from build123d import *

# Parameters (mm, degrees)
F0_W     = 1.6
F0_H     = 10
F1_DEPTH = 8
F2_R     = 2
F3_SIZE  = 3


with BuildPart() as f1:
    # F0 (on Top) → F1 (new body)
    with BuildSketch(Plane.XY):
        Polygon((9.2, 5.6), (9.2, 3.6), (11.2, 5.6), align=None)
        Polygon((7.6, 0), (9.2, 0), (9.2, 3.6), (9.2, 5.6), (9.2, 17.6), (7.6, 17.6), align=None)
        with BuildLine():
            Line((1.6, 0), (0, 0))
            ThreePointArc((0, 0), (4.6, -4.6), (9.2, 0))
            Line((9.2, 0), (7.6, 0))
            ThreePointArc((7.6, 0), (4.6, -3), (1.6, 0))
        make_face()
        with Locations((0.8, 5)):
            Rectangle(F0_W, F0_H)
        Polygon((-8.4, 10), (0, 10), (1.6, 10), (1.6, 11.6), (-8.4, 11.6), align=None)
    extrude(amount=F1_DEPTH)

    # F2
    f2_edges = [f1.edges().sort_by_distance(p)[0] for p in [
        (9.2, 3.6, 4),
    ]]
    fillet(f2_edges, radius=F2_R)

    # F3
    f3_edges = [f1.edges().sort_by_distance(p)[0] for p in [
        (0, 10, 4),
    ]]
    chamfer(f3_edges, length=F3_SIZE)


solid = f1.part
Could you check a few things on this model? Use its own coordinates, in mm. A direction names the side the tool comes from. Give positions to 0.01 mm unless a question says otherwise; leave off trailing zeros. Order: outer loops, then holes, each group sorted by start corner. A loop starts at its lowest first (then second) coordinate and runs counter-clockwise, first axis right, second up.
1. Suppose I cut it at C-C (x = 4.6). Write out the boundary of the cut face in (y, z).
Answers below:
outline: (-4.6, 0) - (-3, 0) - (-3, 8) - (-4.6, 8) - close
2. Thinking about a two-plate mould opening in X: for faces 1 (the flat face through (7.6, 9, 4)), 2 (the flat face through (-2, 9, 4)), 3 (the flat face through (1.6, 6, 4)), 4 (the flat face through (-3, 11.6, 4)), which applies, +X half, -X half, draft (parallel to the pull), parting line (faces both ways), or undercut?
Answers below:
face 1: undercut
face 2: -X half
face 3: undercut
face 4: draft
3. Which directions (+Z, -Z, +X, -X, +Y, -Y) give clear straight access to the entire face, cutting with the end or side of a thin tool? Please do faces 5 (the flat face through (-6, 10, 4)), 6 (the flat face through (10, 5.6, 4)), 7 (the flat face through (8, 17.6, 4)), 8 (the flat face through (9.2, 1, 4)), 9 (the flat face through (-8.4, 11, 4)).
Answers below:
face 5: +Z, -Z, -X, -Y
face 6: +Z, -Z, +X, +Y
face 7: +Z, -Z, +X, -X, +Y
face 8: +Z, -Z, +X, -Y
face 9: +Z, -Z, -X, +Y, -Y
4. Suppose I cut it at A-A (y = 6.25). Write out the boundary of the cut face in (x, z).
Answers below:
outline: (0, 0) - (1.6, 0) - (1.6, 8) - (0, 8) - close; (7.6, 0) - (9.2, 0) - (9.2, 8) - (7.6, 8) - close
5. Suppose I cut it at B-B (z = 0.5). Write out the boundary of the cut face in (x, y).
Answers below:
outline: (-8.4, 10) - (-3, 10) - (0, 7) - (0, 0) arc R4.6 ccw to (9.2, 0) - (9.2, 2.77) arc R2 cw to (9.79, 4.19) - (11.2, 5.6) - (9.2, 5.6) - (9.2, 17.6) - (7.6, 17.6) - (7.6, 0) arc R3 cw to (1.6, 0) - (1.6, 11.6) - (-8.4, 11.6) - close
6. Suppose I cut it at D-D (y = 9). Write out the boundary of the cut face in (x, z), plus the area to 3 significant figures.
Answers below:
outline: (-2, 0) - (1.6, 0) - (1.6, 8) - (-2, 8) - close; (7.6, 0) - (9.2, 0) - (9.2, 8) - (7.6, 8) - close
area: 41.6 mm2
7. For pin 1 (2 mm diameter, centred on y = 5, z = 7, fed in from -X); pin 2 (2.5 mm diameter, centred on y = 10.5, z = 3.5, fed in from +X); pin 3 (2 mm diameter, centred on x = 10.5, z = 2.5, fed in from +Y), each with a flat end and sliding along its axis, tell me the tip position at first contact or that it passes through.
Answers below:
pin 1: stops at x = 0
pin 2: stops at x = 9.2
pin 3: stops at y = 5.6
8. I need wall thicknesses on L1, parallel to X at y = 0.5, z = 5.25; L2, parallel to X at y = 11, z = 6; L3, parallel to Y at x = 4.5, z = 7.25. Which ranges of each line are inside material? Lowest first, please.
Answers below:
L1: x = 0 to 1.6, 7.6 to 9.2
L2: x = -8.4 to 1.6, 7.6 to 9.2
L3: y = -4.6 to -3
